from build123d import *

# Parameters (mm, degrees)
SKETCH1_R           = 2.159
BOSS_EXTRUDE1_DEPTH = 2.286


with BuildPart() as part:
    # Sketch1 → Boss-Extrude1 (new body)
    with BuildSketch(Plane(origin=(0, 0, 0), x_dir=(1, 0, 0), z_dir=(0, 1, 0))):
        Polygon((0, 2.54), (0, 67.056), (2.54, 69.596), (67.056, 69.596), (69.596, 67.056), (69.596, 46.736), (67.056, 44.196), (25.4, 44.196), (25.4, 2.54), (22.86, 0), (2.54, 0), align=None)
        with Locations((12.7, 56.896)):
            Circle(SKETCH1_R, mode=Mode.SUBTRACT)
        with Locations((25.4, 56.896)):
            Circle(SKETCH1_R, mode=Mode.SUBTRACT)
        with Locations((38.1, 56.896)):
            Circle(SKETCH1_R, mode=Mode.SUBTRACT)
        with Locations((50.8, 56.896)):
            Circle(SKETCH1_R, mode=Mode.SUBTRACT)
        with Locations((63.5, 56.896)):
            Circle(SKETCH1_R, mode=Mode.SUBTRACT)
        with Locations((12.7, 44.196)):
            Circle(SKETCH1_R, mode=Mode.SUBTRACT)
        with Locations((12.7, 31.496)):
            Circle(SKETCH1_R, mode=Mode.SUBTRACT)
        with Locations((12.7, 18.796)):
            Circle(SKETCH1_R, mode=Mode.SUBTRACT)
        with Locations((12.7, 6.096)):
            Circle(SKETCH1_R, mode=Mode.SUBTRACT)
    extrude(amount=BOSS_EXTRUDE1_DEPTH)


solid = part.part
CAD build for the part. Positions are in the model's coordinates, mm. A direction names the side the tool comes from. Give positions to 0.01 mm unless a question says otherwise; leave off trailing zeros. Write each loop counter-clockwise with the first axis right and the second up, starting at its lowest first coordinate (ties: lowest second). Pieces come first, ordered by that corner, then holes. Notation, with made-up numbers: M 56,56 L 71,56 A33 ccw 71,95 Z; hole C -1,38 d11. An arc over 180 degrees is marked long. Put each result on its own line as item: value. Start each with the question number.
(1) Band-saw the part on B-B, the plane x = 12.7. Write the cut outline in (y, z) (3 decimals), and give its area (3 significant figures).
(2) Probe L1, parallel to Z at x = 12.7, y = 0.9 (3 decimals); L2, parallel to Z at x = 12.5, y = 0.4; L3, parallel to X at y = 1.25, z = -25. List the from-to ranges inside material, lowest first.
(3) Mould opens along Z. For faces 1 (the face through (28, 2.286, -51)), 2 (the face through (1.29, 1.13, -1.25)), 3 (the face through (37.63, 1.13, -54.79)) say: +Z half, -Z half, draft (parallel to the pull), parting line (faces both ways), or undercut.
(4) Band-saw the part on D-D, the plane y = 0.95. Give the number of separate pieces and of enclosed holes in the cut face, and give its area (3 significant figures).
(5) Flat gauge pins, fed straight in: pin 1 Ø5 at (x, z) = (50.8, -56.896) entering from +Y; pin 2 Ø1.1 at (x, y) = (39.5, 1) entering from +Z; pin 3 Ø0.7 at (y, z) = (0.5, -31) entering from +X. Where does each tip first touch, or does it go through?
(6) Band-saw the part on C-C, the plane z = -45. Write the cut outline in (x, y), and give its area (3 significant figures).
(7) Band-saw the part on A-A, the plane x = 50.8. Write the cut outline in (y, z) (3 decimals).
(8) Which spindle directions (+Z, -Z, +X, -X, +Y, -Y) get a long thin tool onto all of the face, cutting with end or side? Do faces 4 (the face through (47, 1, -44.196)), 5 (the face through (28, 0, -51)). Say none if no direction does.
Response values:
1. outline: M 0,-69.596 L 2.286,-69.596 L 2.286,-59.055 L 0,-59.055 Z; M 0,-54.737 L 2.286,-54.737 L 2.286,-46.355 L 0,-46.355 Z; M 0,-42.037 L 2.286,-42.037 L 2.286,-33.655 L 0,-33.655 Z; M 0,-29.337 L 2.286,-29.337 L 2.286,-20.955 L 0,-20.955 Z; M 0,-16.637 L 2.286,-16.637 L 2.286,-8.255 L 0,-8.255 Z; M 0,-3.937 L 2.286,-3.937 L 2.286,0 L 0,0 Z
1. area: 110 mm2
2. L1: z = -69.596 to -59.055, -54.737 to -46.355, -42.037 to -33.655, -29.337 to -20.955, -16.637 to -8.255, -3.937 to 0
2. L2: z = -69.6 to -59.05, -54.75 to -46.35, -42.05 to -33.65, -29.35 to -20.95, -16.65 to -8.25, -3.95 to 0
2. L3: x = 0 to 25.4
3. face 1: draft
3. face 2: +Z half
3. face 3: undercut
4. separate pieces: 1
4. enclosed holes: 9
4. area: 2,740 mm2
5. pin 1: stops at y = 2.29
5. pin 2: stops at z = -44.2
5. pin 3: stops at x = 25.4
6. outline: M 0,0 L 10.7,0 L 10.7,2.29 L 0,2.29 Z; M 14.7,0 L 67.86,0 L 67.86,2.29 L 14.7,2.29 Z
6. area: 146 mm2
7. outline: M 0,-69.596 L 2.286,-69.596 L 2.286,-59.055 L 0,-59.055 Z; M 0,-54.737 L 2.286,-54.737 L 2.286,-44.196 L 0,-44.196 Z
8. face 4: +Z, +X, +Y, -Y
8. face 5: +Z, -Z, +X, -X, -Y
